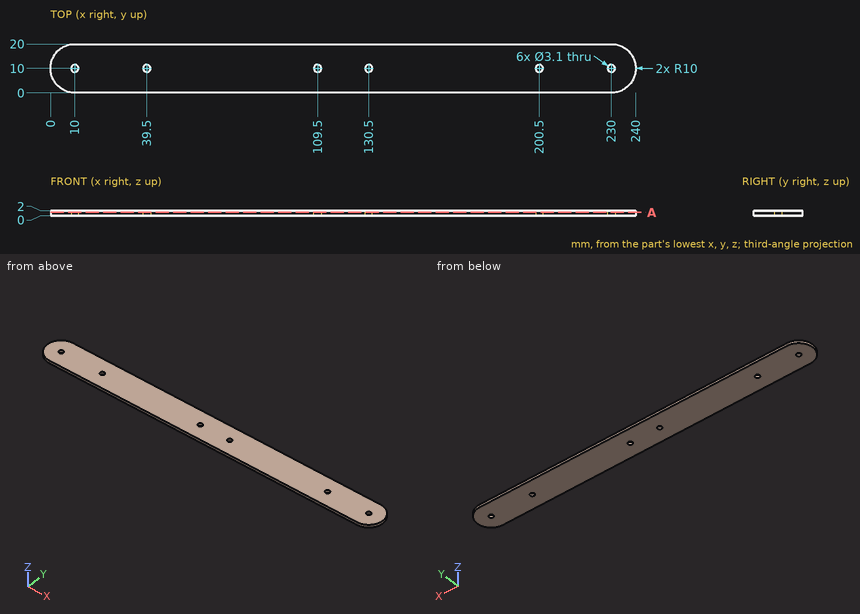
The drawing under review shows one solid part. Ordinate dimensions are in mm from its lowest x, y, z. Round coordinates to 2 decimals unless told otherwise and drop trailing zeros. Order: outer loops, then holes, each group sorted by start corner. A loop starts at its lowest first (then second) coordinate and runs counter-clockwise, first axis right, second up. Notation, with made-up numbers: (44, -23) -> (63, -23) arc R14 ccw to (63, -8) -> close; hole circle Ø1 at (-40, -21). An arc over 180 degrees is marked (long way). Return JSON: item names as keys, results as strings.
1. For L1, parallel to Y at x = 230, z = 1.3; L2, parallel to X at y = 7.25, z = 0.9; L3, parallel to X at y = 4, z = 1.85, list the stretches that pass through material, from the lowest coordinate up. Write a range as [from, to].
Answer block:
{"L1": "y = [0, 8.45], [11.55, 20]", "L2": "x = [0.39, 239.61]", "L3": "x = [2, 238]"}
2. Insertion check: P1, Ø3, axis at x = 109.5, y = 10, coming from the -Z side. The pin has a flat end and moves straight along its axis. Give the tip position at first contact, or say it passes through.
Answer block:
{"P1": "passes through"}
3. Take a section at A-A (z = 1.3). Write out the cut boundary in (x, y).
Answer block:
{"outline": "(10, 0) -> (230, 0) arc R10 ccw to (230, 20) -> (10, 20) arc R10 ccw to start; hole circle Ø3.1 at (10, 10); hole circle Ø3.1 at (39.5, 10); hole circle Ø3.1 at (109.5, 10); hole circle Ø3.1 at (130.5, 10); hole circle Ø3.1 at (200.5, 10); hole circle Ø3.1 at (230, 10)"}
